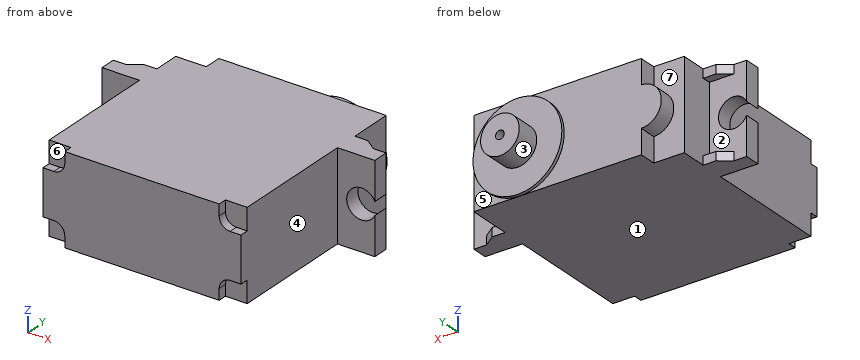
```python
from build123d import *

# Parameters (mm, degrees)
SKETCH1_R               = 2.8194
BOSS_EXTRUDE1_DEPTH     = 3.556
SKETCH2_R               = 6.477
BOSS_EXTRUDE2_DEPTH     = 0.4826
SKETCH3_W               = 28.8544
SKETCH3_H               = 12.954
BOSS_EXTRUDE3_DEPTH     = 29.5148
SKETCH4_R               = 0.635
CUT_EXTRUDE1_DEPTH      = 3.937
SKETCH5_W               = 12.954
SKETCH5_H               = 2.286
BOSS_EXTRUDE4_DEPTH     = 5.4483
BOSS_EXTRUDE5_DEPTH     = 1.27
SKETCH7_R               = 2.159
CUT_EXTRUDE2_DEPTH      = 32.810424981
MIRROR3_COPY_1_DEPTH    = 1.27
CUT_EXTRUDE3_DEPTH      = 2.54
SKETCH10_R              = 1.5875
CUT_EXTRUDE4_DEPTH      = 1.27
MIRROR5_COPY_1_SKETCH_R = 1.5875
MIRROR5_COPY_1_DEPTH    = 1.27


with BuildPart() as part:
    # Sketch1 → Boss-Extrude1 (new body)
    with BuildSketch(Plane(origin=(0, 0, 0), x_dir=(1, 0, 0), z_dir=(0, 1, 0))):
        with Locations(Location((0, 0, 0), (0, 0, 270))):
            Circle(SKETCH1_R)
    extrude(amount=BOSS_EXTRUDE1_DEPTH)

    # Sketch2 → Boss-Extrude2 (add)
    with BuildSketch(Plane(origin=(0, 0, 0), x_dir=(-1, 0, 0), z_dir=(0, -1, 0))):
        with Locations(Location((0, 0, 0), (0, 0, 270))):
            Circle(SKETCH2_R)
    extrude(amount=BOSS_EXTRUDE2_DEPTH)

    # Sketch3 → Boss-Extrude3 (add)
    with BuildSketch(Plane(origin=(0, -0.4826, 0), x_dir=(-1, 0, 0), z_dir=(0, -1, 0))):
        with Locations((7.7216, 0)):
            Rectangle(SKETCH3_W, SKETCH3_H)
    extrude(amount=BOSS_EXTRUDE3_DEPTH)

    # Sketch4 → Cut-Extrude1 (cut)
    with BuildSketch(Plane(origin=(0, 3.556, 0), x_dir=(1, 0, 0), z_dir=(0, 1, 0))):
        with Locations(Location((0, 0, 0), (0, 0, 270))):
            Circle(SKETCH4_R)
    extrude(amount=-CUT_EXTRUDE1_DEPTH, mode=Mode.SUBTRACT)

    # Sketch5 → Boss-Extrude4 (add)
    with BuildSketch(Plane(origin=(6.7056, 0, 0), x_dir=(0, 0, -1), z_dir=(1, 0, 0))):
        with Locations((0, -9.2456)):
            Rectangle(SKETCH5_W, SKETCH5_H)
    boss_extrude4 = extrude(amount=BOSS_EXTRUDE4_DEPTH)

    # Sketch6 → Boss-Extrude5 (add)
    with BuildSketch(Plane.XY.offset(6.477)):
        Polygon((6.7056, -8.1026), (10.2997, -8.1026), (8.5979, -6.866466582), (6.7056, -6.866466582), align=None)
    boss_extrude5 = extrude(amount=-BOSS_EXTRUDE5_DEPTH)

    # Mirror1: Boss-Extrude5 across plane
    add(boss_extrude5.mirror(Plane.XY))

    # Sketch7 → Cut-Extrude2 (cut, through all)
    with BuildSketch(Plane(origin=(0, -8.1026, 0), x_dir=(1, 0, 0), z_dir=(0, 1, 0))):
        with Locations((10.2108, 0)):
            Circle(SKETCH7_R)
    cut_extrude2 = extrude(amount=-CUT_EXTRUDE2_DEPTH, mode=Mode.SUBTRACT)

    # Mirror3: Boss-Extrude4, Boss-Extrude5, Cut-Extrude2 across plane
    add(boss_extrude4.mirror(Plane(origin=(-7.7216, 0, 0), x_dir=(0, 0, 1), z_dir=(1, 0, 0))))
    add(boss_extrude5.mirror(Plane(origin=(-7.7216, 0, 0), x_dir=(0, 0, 1), z_dir=(1, 0, 0))))
    add(cut_extrude2.mirror(Plane(origin=(-7.7216, 0, 0), x_dir=(0, 0, 1), z_dir=(1, 0, 0))), mode=Mode.SUBTRACT)

    # Mirror3 copy 1 sketch → Mirror3 copy 1 (add)
    with BuildSketch(Plane(origin=(-15.4432, 0, -6.477), x_dir=(-1, 0, 0), z_dir=(0, 0, -1))):
        Polygon((6.7056, -8.1026), (10.2997, -8.1026), (8.5979, -6.866466582), (6.7056, -6.866466582), align=None)
    extrude(amount=-MIRROR3_COPY_1_DEPTH)

    # Sketch9 → Cut-Extrude3 (cut)
    with BuildSketch(Plane(origin=(0, -0.4826, 0), x_dir=(1, 0, 0), z_dir=(0, 1, 0))):
        with BuildLine():
            Line((-22.1488, 6.477), (-22.1488, -6.477))
            Line((-22.1488, -6.477), (-17.7038, -6.477))
            Line((-17.7038, -6.477), (-17.7038, -2.921))
            ThreePointArc((-17.7038, -2.921), (-20.6248, 0), (-17.7038, 2.921))
            Line((-17.7038, 2.921), (-17.7038, 6.477))
            Line((-17.7038, 6.477), (-22.1488, 6.477))
        make_face()
    extrude(amount=-CUT_EXTRUDE3_DEPTH, mode=Mode.SUBTRACT)

    # Sketch10 → Cut-Extrude4 (cut)
    with BuildSketch(Plane(origin=(0, -29.9974, 0), x_dir=(-1, 0, 0), z_dir=(0, -1, 0))):
        with Locations((20.5613, 4.8895)):
            Circle(SKETCH10_R)
        with BuildLine():
            Line((22.1488, 6.477), (20.5613, 6.477))
            ThreePointArc((20.5613, 6.477), (21.683832015, 6.012032015), (22.1488, 4.8895))
            Line((22.1488, 4.8895), (22.1488, 6.477))
        make_face()
        with BuildLine():
            ThreePointArc((18.9738, 4.8895), (19.438767985, 6.012032015), (20.5613, 6.477))
            Line((20.5613, 6.477), (18.9738, 6.477))
            Line((18.9738, 6.477), (18.9738, 4.8895))
        make_face()
        with BuildLine():
            Line((22.1488, 3.302), (22.1488, 4.8895))
            ThreePointArc((22.1488, 4.8895), (21.683832015, 3.766967985), (20.5613, 3.302))
            Line((20.5613, 3.302), (22.1488, 3.302))
        make_face()
    cut_extrude4 = extrude(amount=-CUT_EXTRUDE4_DEPTH, mode=Mode.SUBTRACT)

    # Mirror4: Cut-Extrude4 across plane
    add(cut_extrude4.mirror(Plane.XY), mode=Mode.SUBTRACT)

    # Mirror5: Cut-Extrude4 across plane
    add(cut_extrude4.mirror(Plane(origin=(-7.7216, 0, 0), x_dir=(0, 0, 1), z_dir=(1, 0, 0))), mode=Mode.SUBTRACT)

    # Mirror5 copy 1 sketch → Mirror5 copy 1 (cut)
    with BuildSketch(Plane(origin=(-15.4432, -29.9974, 0), x_dir=(1, 0, 0), z_dir=(0, -1, 0))):
        with Locations((20.5613, 4.8895)):
            Circle(MIRROR5_COPY_1_SKETCH_R)
        with BuildLine():
            Line((22.1488, 6.477), (20.5613, 6.477))
            ThreePointArc((20.5613, 6.477), (21.683832015, 6.012032015), (22.1488, 4.8895))
            Line((22.1488, 4.8895), (22.1488, 6.477))
        make_face()
        with BuildLine():
            ThreePointArc((18.9738, 4.8895), (19.438767985, 6.012032015), (20.5613, 6.477))
            Line((20.5613, 6.477), (18.9738, 6.477))
            Line((18.9738, 6.477), (18.9738, 4.8895))
        make_face()
        with BuildLine():
            Line((22.1488, 3.302), (22.1488, 4.8895))
            ThreePointArc((22.1488, 4.8895), (21.683832015, 3.766967985), (20.5613, 3.302))
            Line((20.5613, 3.302), (22.1488, 3.302))
        make_face()
    extrude(amount=-MIRROR5_COPY_1_DEPTH, mode=Mode.SUBTRACT)


solid = part.part
```
For this review, take the finished solid that the model builds, in its own axes (mm). Face numbers are marked on the shaded views. A direction names the side the tool comes from. Round coordinates to 2 decimals unless told otherwise and drop trailing zeros. Write each loop counter-clockwise with the first axis right and the second up, starting at its lowest first coordinate (ties: lowest second). Pieces come first, ordered by that corner, then holes. Notation, with made-up numbers: (24.25, -33) - (38.25, -33) arc R27 cw to (38.25, 6) - close; hole circle Ø5 at (-34.5, -19). An arc over 180 degrees is marked (long way). Put each result on its own line as item: value.
Q1. We need section C-C (y = -2.5). Give the boundary of the cut face in (x, z), and give its area (3 significant figures).
Solved:
outline: (-17.7, -6.48) - (6.71, -6.48) - (6.71, 6.48) - (-17.7, 6.48) - (-17.7, 2.92) arc R2.92 ccw to (-17.7, -2.92) - close
area: 330 mm2
Q2. Wall thickness on probe 1 along Z at (x, y) = (8.5, -8); probe 2 along Y at (x, z) = (-21, 0.5); probe 3 along Y at (x, z) = (2.5, 5): over which ranges is each line inside the solid? List them lowest first.
Solved:
probe 1: z = -6.48 to -5.21, 5.21 to 6.48
probe 2: y = -30 to -3.02
probe 3: y = -30 to 0
Q3. We need section A-A (z = 1.5). Count the separate pieces of the cut face and the enclosed holes in it, and give its area (3 significant figures).
Solved:
separate pieces: 3
enclosed holes: 0
area: 880 mm2
Q4. We need section D-D (x = -12). Give the boundary of the cut face in (y, z).
Solved:
outline: (-30, -6.48) - (-0.48, -6.48) - (-0.48, 6.48) - (-30, 6.48) - close
Q5. We need section B-B (y = 1). Give the boundary of the cut face in (x, z) (3 decimals), and give its area (3 significant figures).
Solved:
outline: circle Ø5.639 at (0, 0); hole circle Ø1.27 at (0, 0)
area: 23.7 mm2
Q6. Mouldability with a two-part tool opening along Z and no side actions: class the marked faces 1, 2 and 3 as released by +Z, released by -Z, zero draft, split by the parting line, or undercut.
Solved:
face 1: released by -Z
face 2: undercut
face 3: split by the parting line
Q7. Insertion check: pin 1 Ø0.6 at (x, z) = (-23, 6) entering from +Y; pin 2 Ø4 at (y, z) = (-21, 1) entering from -X; pin 3 Ø5 at (x, z) = (-20.5, -1) entering from +Y. Each pin has a flat end and moves straight along its axis. Give the tip position at first contact, or say it passes through.
Solved:
pin 1: stops at y = -6.87
pin 2: stops at x = -22.15
pin 3: stops at y = -0.48
Q8. Machinability: for the marked faces 4, 5, 6 and 7, which of the approach directions +Z, -Z, +X, -X, +Y, -Y give a long, thin tool a straight path to every point of the face, cutting with its end or side? Answer none if there is none.
Solved:
face 4: +Z, -Z, +X, -Y
face 5: +X, +Y
face 6: +Z, -X, -Y
face 7: -X, +Y
